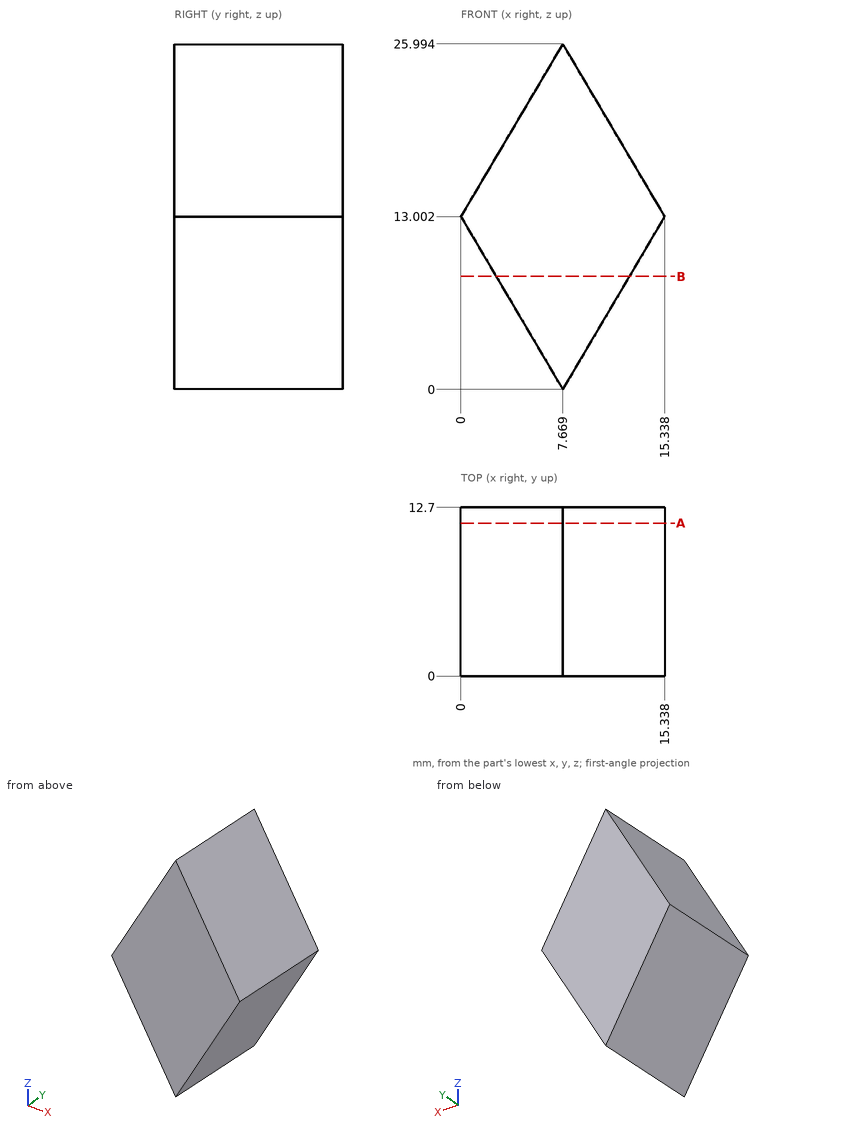
Answer from the drawing. Dimensions are ordinates in mm from the lowest x, y and z of the part. Round coordinates to 2 decimals unless told otherwise and drop trailing zeros. Order: outer loops, then holes, each group sorted by start corner. A loop starts at its lowest first (then second) coordinate and runs counter-clockwise, first axis right, second up. Notation, with made-up numbers: (26.5, 67) -> (39.5, 67) arc R26 cw to (39.5, 91) -> close; hole circle Ø6 at (41.25, 10). An arc over 180 degrees is marked (long way). Answer as CSV lines item,"result".
Q1. Consider line 1 (Z direction, x = 4, y = 5.5) (1 decimal); line 2 (Z direction, x = 7.5, y = 1.25) (1 decimal); line 3 (X direction, y = 2.25, z = 21) (1 decimal). Determine where each line is inside the solid, lowest interval first. Write a range as from..to.
Computed values:
line 1,"z = 6.2..19.8"
line 2,"z = 0.3..25.7"
line 3,"x = 4.7..10.6"
Q2. Given pin 1 (3 mm diameter, centred on y = 9, z = 18.5, fed in from +X); pin 2 (1.5 mm diameter, centred on y = 3, z = 13.5, fed in from +X); pin 3 (4 mm diameter, centred on x = 11, y = 10.5, fed in from +Z); pin 4 (4 mm diameter, centred on x = 6, y = 10.5, fed in from -Z), each flat-ended and moving along its own axis, determine where each tip first touches the part or whether it passes through.
Computed values:
pin 1,"stops at x = 12.98"
pin 2,"stops at x = 15.34"
pin 3,"stops at z = 23.74"
pin 4,"stops at z = 0"
Q3. A cutting plane is placed at A-A on y = 11.5. Determine the outline of the cut face in (x, z).
Computed values:
outline,"(0, 13) -> (7.67, 0) -> (15.34, 13) -> (7.67, 25.99) -> close"
Q4. A cutting plane is placed at B-B on z = 8.5. Determine the outline of the cut face in (x, y) (1 decimal).
Computed values:
outline,"(2.7, 0) -> (12.7, 0) -> (12.7, 12.7) -> (2.7, 12.7) -> close"
